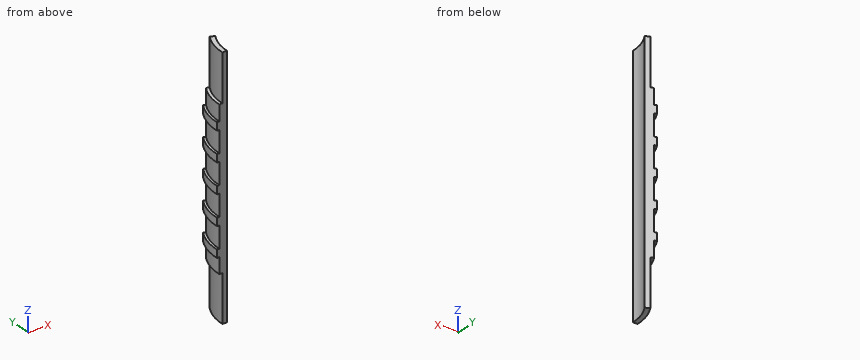
Autodesk Inventor part; units mm, degrees
ref_plane "YZ Plane" through (0, 0, 0) normal (1, 0, 0) x (0, 1, 0)
ref_plane "XZ Plane" through (0, 0, 0) normal (0, 1, 0) x (-1, 0, 0)
ref_plane "XY Plane" through (0, 0, 0) normal (0, 0, 1) x (1, 0, 0)
sketch "Skizze1" plane through (0, 0, 0) normal (0, 0, 1) x (1, 0, 0)
  arc A0 (-15, 25.9808) -> (-30, 0) centre (0, 0) ccw
  line L0 (-15, 25.9808) -> (-16.8174, 28.3932)
  line L1 (-30, 0) -> (-33, 0)
  arc A1 (-16.8174, 28.3932) -> (-33, 0) centre (0, 0) ccw
extrude "Teil B1" add sketch "Skizze1" along normal blind 30
sketch "Skizze2" plane through (0, 0, 30) normal (0, 0, 1) x (1, 0, 0)
  arc A0 (-15, 25.9808) -> (-30, 0) centre (0, 0) ccw
  line L0 (-33, 0) -> (-30, 0)
  arc A1 (-15, 25.9808) -> (-30, 0) centre (0, 0) ccw
  arc A2 (-18.0278, 30) -> (-35, 0) centre (0, 0) ccw
  line L1 (-30, 0) -> (-35, 0)
  line L2 (-15, 25.9808) -> (-18.0278, 30)
  line L3 (-15, 25.9808) -> (-16.8174, 28.3932)
  dimension "d6" = 70
extrude "Teil C1" add sketch "Skizze2" along normal blind 10
sketch "Skizze3" plane through (0, 0, 40) normal (0, 0, 1) x (1, 0, 0)
  arc A0 (-15, 25.9808) -> (-30, 0) centre (0, 0) ccw
  line L0 (-33, 0) -> (-30, 0)
  arc A1 (-15, 25.9808) -> (-30, 0) centre (0, 0) ccw
  arc A2 (-18.935, 31.2044) -> (-36.5, 0) centre (0, 0) ccw
  line L1 (-30, 0) -> (-36.5, 0)
  line L2 (-15, 25.9808) -> (-16.8174, 28.3932)
  line L3 (-15, 25.9808) -> (-18.935, 31.2044)
  dimension "d9" = 73
extrude "Teil D1" add sketch "Skizze3" along normal blind 5
sketch "Skizze4" plane through (0, 0, 45) normal (0, 0, 1) x (1, 0, 0)
  arc A0 (-18.0278, 30) -> (-35, 0) centre (0, 0) ccw
  arc A1 (-15, 25.9808) -> (-30, 0) centre (0, 0) ccw
  arc A2 (-15, 25.9808) -> (-30, 0) centre (0, 0) ccw
  line L0 (-16.8174, 28.3932) -> (-18.0278, 30)
  line L1 (-15, 25.9808) -> (-18.0278, 30)
  line L2 (-36.5, 0) -> (-35, 0)
  line L3 (-30, 0) -> (-35, 0)
extrude "Teil E1" add sketch "Skizze4" along normal blind 13.75
sketch "Skizze5" plane through (0, 0, 58.75) normal (0, 0, 1) x (1, 0, 0)
  arc A0 (-15, 25.9808) -> (-30, 0) centre (0, 0) ccw
  arc A1 (-15, 25.9808) -> (-30, 0) centre (0, 0) ccw
  arc A2 (-18.935, 31.2044) -> (-36.5, 0) centre (0, 0) ccw
  line L0 (-36.5, 0) -> (-35, 0)
  arc A3 (-18.935, 31.2044) -> (-36.5, 0) centre (0, 0) ccw
  line L1 (-33, 0) -> (-30, 0)
  line L2 (-36.5, 0) -> (-30, 0)
  line L3 (-15, 25.9808) -> (-18.935, 31.2044)
  point P0 (-15, 25.9808)
extrude "Teil D2" add sketch "Skizze5" along normal blind 5
sketch "Skizze6" plane through (0, 0, 63.75) normal (0, 0, 1) x (1, 0, 0)
  line L0 (-33, 0) -> (-30, 0)
  arc A0 (-15, 25.9808) -> (-30, 0) centre (0, 0) ccw
  arc A1 (-18.0278, 30) -> (-35, 0) centre (0, 0) ccw
  arc A2 (-18.0278, 30) -> (-35, 0) centre (0, 0) ccw
  line L1 (-36.5, 0) -> (-35, 0)
  line L2 (-35, 0) -> (-30, 0)
  line L3 (-15, 25.9808) -> (-18.0278, 30)
  line L4 (-15, 25.9808) -> (-16.8174, 28.3932)
extrude "Extrusion6" add sketch "Skizze6" along normal blind 13.75
sketch "Skizze7" plane through (0, 0, 77.5) normal (0, 0, 1) x (1, 0, 0)
  arc A0 (-15, 25.9808) -> (-30, 0) centre (0, 0) ccw
  line L0 (-33, 0) -> (-30, 0)
  arc A1 (-15, 25.9808) -> (-30, 0) centre (0, 0) ccw
  line L1 (-18.0278, 30) -> (-18.935, 31.2044)
  line L2 (-36.5, 0) -> (-35, 0)
  arc A2 (-18.935, 31.2044) -> (-36.5, 0) centre (0, 0) ccw
  line L3 (-36.5, 0) -> (-30, 0)
  line L4 (-15, 25.9808) -> (-16.8174, 28.3932)
  line L5 (-18.935, 31.2044) -> (-15, 25.9808)
extrude "Extrusion7" add sketch "Skizze7" along normal blind 2.5
mirror "Spiegeln1" about plane through (-25.75, 15.6022, 80) normal (0, 0, 1)
sketch "Skizze8" plane through (-33, 0, 160) normal (0, 0, 1) x (1, 0, 0)
  arc A0 (18, 25.9808) -> (3, 0) centre (33, 0) ccw
  line L0 (3, 0) -> (13, 17.3205)
  line L1 (13, 17.3205) -> (4.1881, 22.4081)
  arc A1 (14.065, 31.2044) -> (-3.5, 0) centre (33, 0) ccw
  arc A2 (18, 25.9808) -> (9.8826, 19.1203) centre (33, 0) ccw
  arc A3 (14.065, 31.2044) -> (4.1881, 22.4081) centre (33, 0) ccw
  line L2 (14.065, 31.2044) -> (18, 25.9808)
  dimension "d21" = 20
extrude "Extrusion8" cut sketch "Skizze8" against normal through all contours A0 L1 A1 L2
sketch "Skizze9" plane through (-33, 0, 160) normal (0, 0, 1) x (1, 0, 0)
  line L0 (0, 0) -> (3, 0)
  arc A0 (9.8826, 19.1203) -> (3, 0) centre (33, 0) ccw
  arc A1 (3, 0) -> (7.8167, 16.3034) centre (-4.5602, 11.0968) ccw
  line L1 (7.8167, 16.3034) -> (1.9088, 19.1203)
  arc A2 (4.1881, 22.4081) -> (-3.5, 0) centre (33, 0) ccw
  line L2 (4.1881, 22.4081) -> (9.8826, 19.1203)
  arc A3 (4.1881, 22.4081) -> (1.9088, 19.1203) centre (33, 0) ccw
  arc A4 (9.8826, 19.1203) -> (7.8167, 16.3034) centre (33, 0) ccw
  dimension "d24" = 17
extrude "Extrusion9" cut sketch "Skizze9" against normal through all contours A0 L1 A2 L2
properties part number "Bumper_V1"
Build history of the part. All positions in model axes, mm. Give positions to 0.01 mm unless a question says otherwise; leave off trailing zeros. Loops run counter-clockwise (first coordinate to the right, second up) from the corner with the lowest first, then second, coordinate; pieces in that order, holes last. Notation, with made-up numbers: (-34, 86) - (13, 86) arc R17 ccw to (13, 114) - close; hole circle Ø9 at (72, -9.75). An arc over 180 degrees is marked (long way). Write item = value, one per line. Start each with the question number.
1) Band-saw the part on C-C on y = 13. Give the cut face in (x, z).
2) Drop flat-ended pins along their axis: pin 1 Ø3.5 at (x, y) = (-33, 12.5) entering from -Z; pin 2 Ø4 at (x, y) = (-32, 16) entering from +Z; pin 3 Ø5 at (y, z) = (7, 118.5) entering from -X. Give the stop position or say it passes through.
3) Band-saw the part on B-B on z = 20.5. Give the cut face in (x, y).
4) Probe probe 1 along Z at (x, y) = (-35.75, 5); probe 2 along Z at (x, y) = (-30.75, 15.75); probe 3 along X at (y, z) = (11, 115.5). List the from-to ranges inside material, lowest first. Write a range as from..to.
5) Band-saw the part on D-D on z = 91. Give the cut face in (x, y), plus the area to 3 significant figures.
6) Band-saw the part on A-A on y = 1.5. Give the cut face in (x, z).
Final values:
q1.outline = (-34.11, 40) - (-32.5, 40) - (-32.5, 30) - (-30.33, 30) - (-30.33, 0) - (-27.04, 0) - (-27.04, 160) - (-30.33, 160) - (-30.33, 130) - (-32.5, 130) - (-32.5, 120) - (-34.11, 120) - (-34.11, 115) - (-32.5, 115) - (-32.5, 101.25) - (-34.11, 101.25) - (-34.11, 96.25) - (-32.5, 96.25) - (-32.5, 82.5) - (-34.11, 82.5) - (-34.11, 77.5) - (-32.5, 77.5) - (-32.5, 63.75) - (-34.11, 63.75) - (-34.11, 58.75) - (-32.5, 58.75) - (-32.5, 45) - (-34.11, 45) - close
q2.pin_1 = 30
q2.pin_2 = 130
q2.pin_3 = -36.22
q3.outline = (-33, 0) - (-30, 0) arc R30 cw to (-25.18, 16.3) - (-27.91, 17.6) arc R33 ccw to start
q4.probe_1 = 40..45, 58.75..63.75, 77.5..82.5, 96.25..101.25, 115..120
q4.probe_2 = 30..130
q4.probe_3 = -34.8..-27.91
q5.outline = (-35, 0) - (-30, 0) arc R30 cw to (-25.18, 16.3) - (-29.73, 18.47) arc R35 ccw to start
q5.area = 91.7 mm²
q6.outline = (-36.47, 40) - (-34.97, 40) - (-34.97, 30) - (-32.97, 30) - (-32.97, 0) - (-29.96, 0) - (-29.96, 160) - (-32.97, 160) - (-32.97, 130) - (-34.97, 130) - (-34.97, 120) - (-36.47, 120) - (-36.47, 115) - (-34.97, 115) - (-34.97, 101.25) - (-36.47, 101.25) - (-36.47, 96.25) - (-34.97, 96.25) - (-34.97, 82.5) - (-36.47, 82.5) - (-36.47, 77.5) - (-34.97, 77.5) - (-34.97, 63.75) - (-36.47, 63.75) - (-36.47, 58.75) - (-34.97, 58.75) - (-34.97, 45) - (-36.47, 45) - close
